Design review of the part built by this model. Coordinates are the model's own, in mm. A direction names the side the tool comes from. Coordinates: 2 decimals unless noted, no trailing zeros. Loops run counter-clockwise (first coordinate to the right, second up) from the corner with the lowest first, then second, coordinate; pieces in that order, holes last. Notation, with made-up numbers: (45, 73) - (104, 73) arc R26 ccw to (104, 94) - close; hole circle Ø7 at (57.5, 45). An arc over 180 degrees is marked (long way). Use one line per item in the form item = value. Start each with the question number.
(1) For L1, parallel to Y at x = -6, z = 7.5; L2, parallel to Z at x = 0, y = -9.25; L3, parallel to X at y = -1.75, z = 13.75, list the stretches that pass through material, from the lowest coordinate up.
(2) Tool access review of faces 1 (the face through (0, -1, -3)), 2 (the face through (0.92, -6.44, 10.67)): name each direction out of +Z, -Z, +X, -X, +Y, -Y from which nothing blocks a thin tool from reaching the whole face with its end or side.
(3) Add section B-B (x = 10). State the section outline as (y, z) points, plus the area to 3 significant figures.
(4) Add section D-D (x = -6). State the section outline as (y, z) points, plus the area to 3 significant figures.
(5) Clearance check with flat-ended pins moving along their axes: pin 1 Ø5 at (x, y) = (-1.5, -8.5) entering from -Z; pin 2 Ø3 at (x, y) = (-4, -7.5) entering from -Z. State where each tip first meets the part, or that it passes through.
(6) Add section C-C (y = -3). State the section outline as (x, z) points.
(7) Add section A-A (z = 11.75). State the section outline as (x, y) points.
```python
from build123d import *

# Parameters (mm, degrees)
F1_DEPTH = 2
F2_R     = 2
F3_DEPTH = 9
F4_R     = 3
F5_DEPTH = 2


with BuildPart() as f1:
    # F0 (on Front) → F1 (new body)
    with BuildSketch(Plane.XZ):
        with BuildLine():
            Line((-11.4086838439, 16.9650800526), (-3, 0))
            Line((-3, 0), (3, 0))
            Line((3, 0), (11.4086838439, 16.9650800526))
            ThreePointArc((11.4086838439, 16.9650800526), (5.9637128105, 19.5552074332), (0, 20.444363728))
            ThreePointArc((0, 20.444363728), (-5.9637128105, 19.5552074332), (-11.4086838439, 16.9650800526))
        make_face()
    extrude(amount=F1_DEPTH)

    # F2 (on face) → F3 (join)
    with BuildSketch(Plane.XZ.offset(2)):
        with Locations((0, 12.444363728)):
            Circle(F2_R)
    extrude(amount=F3_DEPTH)

    # F4 (on Front) → F5 (join)
    with BuildSketch(Plane.XZ):
        Circle(F4_R)
    extrude(amount=F5_DEPTH)


solid = f1.part
```
Computed values:
q1.L1 = -2 to 0
q1.L2 = 10.44 to 14.44
q1.L3 = -9.82 to 9.82
q2.face_1 = -Z, +Y, -Y
q2.face_2 = -Y
q3.outline = (-2, 14.12) - (0, 14.12) - (0, 17.83) - (-2, 17.83) - close
q3.area = 7.42 mm^2
q4.outline = (-2, 6.05) - (0, 6.05) - (0, 19.54) - (-2, 19.54) - close
q4.area = 27.0 mm^2
q5.pin_1 = 10.44
q5.pin_2 = through
q6.outline = circle Ø4 at (0, 12.44)
q7.outline = (-8.82, -2) - (-1.88, -2) - (-1.88, -11) - (1.88, -11) - (1.88, -2) - (8.82, -2) - (8.82, 0) - (-8.82, 0) - close
